Autodesk Inventor part; units mm, degrees
ref_plane "YZ Plane" through (0, 0, 0) normal (1, 0, 0) x (0, 1, 0)
ref_plane "XZ Plane" through (0, 0, 0) normal (0, 1, 0) x (-1, 0, 0)
ref_plane "XY Plane" through (0, 0, 0) normal (0, 0, 1) x (1, 0, 0)
sketch "Skizze1" plane through (0, 0, 0) normal (0, 0, 1) x (1, 0, 0)
  line L0 (-18.7799, 0) -> (18.7799, 0)
  line L1 (0, -24.3799) -> (0, 24.3799)
  line L2 (-11, -17) -> (11, -17)
  line L3 (13, -15) -> (13, 15)
  line L4 (11, 17) -> (-11, 17)
  line L5 (-13, 15) -> (-13, -15)
  line L6 (-13, -17) -> (13, 17) construction
  line L7 (13, -17) -> (-13, 17) construction
  arc A0 (-11, 17) -> (-13, 15) centre (-11, 15) ccw
  arc A1 (13, 15) -> (11, 17) centre (11, 15) ccw
  arc A2 (11, -17) -> (13, -15) centre (11, -15) ccw
  arc A3 (-13, -15) -> (-11, -17) centre (-11, -15) ccw
  point P0 (0, 0)
  dimension "d0" = 26
  dimension "d1" = 34
  dimension "d2" = 2
extrude "Extrusion1" add sketch "Skizze1" against normal blind 2
sketch "Skizze2" plane through (0, 0, 0) normal (0, 0, 1) x (1, 0, 0)
  line L0 (13, -15) -> (13, 15)
  arc A0 (13, 15) -> (11, 17) centre (11, 15) ccw
  line L1 (11, 17) -> (-11, 17)
  arc A1 (-11, 17) -> (-13, 15) centre (-11, 15) ccw
  line L2 (-13, 15) -> (-13, -15)
  arc A2 (-13, -15) -> (-11, -17) centre (-11, -15) ccw
  line L3 (-11, -17) -> (11, -17)
  arc A3 (11, -17) -> (13, -15) centre (11, -15) ccw
  line L4 (-18.7799, 0) -> (18.7799, 0)
  line L5 (0, -24.3799) -> (0, 24.3799)
  line L6 (-5, 4) -> (5, 4)
  line L7 (5, 4) -> (5, -6)
  line L8 (5, -6) -> (-5, -6)
  line L9 (-5, -6) -> (-5, 4)
  arc A4 (5, 4) -> (-5, 4) centre (0, 4) ccw
  point P0 (0, 0)
  dimension "d5" = 10
  dimension "d6" = 10
  dimension "d7" = 11
  dimension "d8" = 5
extrude "Extrusion2" cut sketch "Skizze2" against normal blind 2 contours L7 L8 L5 L4 | L4 L5 L6 L7 | L5 L8 L9 L4 | L4 L9 L6 L5 | L6 L5 A4 | L6 A4 L5
sketch "Skizze3" plane through (0, 0, 0) normal (0, 0, 1) x (1, 0, 0)
  line L0 (5, 4) -> (5, -6)
  line L1 (5, -6) -> (-5, -6)
  line L2 (-5, -6) -> (-5, 4)
  arc A0 (5, 4) -> (-5, 4) centre (0, 4) ccw
  line L3 (13, -15) -> (13, 15)
  arc A1 (13, 15) -> (11, 17) centre (11, 15) ccw
  line L4 (11, 17) -> (-11, 17)
  arc A2 (-11, 17) -> (-13, 15) centre (-11, 15) ccw
  line L5 (-13, 15) -> (-13, -15)
  arc A3 (-13, -15) -> (-11, -17) centre (-11, -15) ccw
  line L6 (-11, -17) -> (11, -17)
  arc A4 (11, -17) -> (13, -15) centre (11, -15) ccw
  line L7 (-18.7799, 0) -> (18.7799, 0)
  line L8 (0, -24.3799) -> (0, 24.3799)
  point P0 (0, 0)
  point P1 (0, -12)
  point P2 (0, 13)
  dimension "d11" = 25
  dimension "d12" = 5
hole "Bohrung1" at (0, -12, 0) at (0, 13, 0) direction (0, 0, -1) diameter 3.5 end through all countersink diameter 7 countersink angle 90
properties part number "Rückwand Deckplatte" material "PVC, hart"
The model under review builds one solid part; all positions refer to its coordinate system, in mm. A direction names the side the tool comes from. Round coordinates to 2 decimals unless told otherwise and drop trailing zeros. Loops run counter-clockwise (first coordinate to the right, second up) from the corner with the lowest first, then second, coordinate; pieces in that order, holes last. Notation, with made-up numbers: (81.5, 70) - (127.5, 70) arc R27 ccw to (127.5, 108) - close; hole circle Ø8 at (-33, 67.5). An arc over 180 degrees is marked (long way). Use CSV: the item, a comma, the result in double quotes.
(1) The part is to be moulded in two halves that separate along X. For faces 1 (the cylindrical face through (-12.4, 16.43, -0.99)), 2 (the cylindrical face through (12.43, 16.4, -0.99)), 3 (the conical face through (0.1, -10.1, -1.6)), say which applies: pulls with the +X half, pulls with the -X half, needs draft (parallel to the pull), parting line crosses it, or undercut.
Working result:
face 1,"pulls with the -X half"
face 2,"pulls with the +X half"
face 3,"undercut"
(2) Take a section at C-C, the plane z = -0.55. Give the boundary of the cut face in (x, y).
Working result:
outline,"(-13, -15) arc R2 ccw to (-11, -17) - (11, -17) arc R2 ccw to (13, -15) - (13, 15) arc R2 ccw to (11, 17) - (-11, 17) arc R2 ccw to (-13, 15) - close; hole (-5, -6) - (5, -6) - (5, 4) arc R5 ccw to (-5, 4) - close; hole circle Ø5.9 at (0, -12); hole circle Ø5.9 at (0, 13)"
(3) Machinability: for faces 4 (the flat face through (-13, 0, -1)), 5 (the cylindrical face through (0, 9, -1)), which of the approach directions +Z, -Z, +X, -X, +Y, -Y give a long, thin tool a straight path to every point of the face, cutting with its end or side? Answer none if there is none.
Working result:
face 4,"+Z, -Z, -X, +Y, -Y"
face 5,"+Z, -Z"
(4) Take a section at B-B, the plane x = 0. Give the boundary of the cut face in (y, z), plus the area to 3 significant figures.
Working result:
outline,"(-17, -2) - (-13.75, -2) - (-13.75, -1.75) - (-15.5, 0) - (-17, 0) - close; (-10.25, -2) - (-6, -2) - (-6, 0) - (-8.5, 0) - (-10.25, -1.75) - close; (9, -2) - (11.25, -2) - (11.25, -1.75) - (9.5, 0) - (9, 0) - close; (14.75, -2) - (17, -2) - (17, 0) - (16.5, 0) - (14.75, -1.75) - close"
area,"17.9 mm^2"
(5) Take a section at A-A, the plane y = 8. Give the boundary of the cut face in (x, z), plus the area to 3 significant figures.
Working result:
outline,"(-13, -2) - (-3, -2) - (-3, 0) - (-13, 0) - close; (3, -2) - (13, -2) - (13, 0) - (3, 0) - close"
area,"40.0 mm^2"
(6) Clearance check with a flat-ended pin moving along its axis: P1, Ø1.5, axis at x = -1.5, y = 11.5, coming from the +Z side. State where the tip first meets the part, or that it passes through.
Working result:
P1,"stops at z = -0.63"
(7) Take a section at D-D, the plane y = -2. Give the boundary of the cut face in (x, z).
Working result:
outline,"(-13, -2) - (-5, -2) - (-5, 0) - (-13, 0) - close; (5, -2) - (13, -2) - (13, 0) - (5, 0) - close"
(8) For line 1 (Y direction, x = 0, z = -1.85); line 2 (X direction, y = 13, z = -1.85), list the stretches that pass through material, from the lowest coordinate up.
Working result:
line 1,"y = -17 to -13.75, -10.25 to -6, 9 to 11.25, 14.75 to 17"
line 2,"x = -13 to -1.75, 1.75 to 13"
